from build123d import *

# Parameters (mm, degrees)
SKETCH_R     = 9
PAD_DEPTH    = 20
SKETCH002_W  = 12
SKETCH002_H  = 12
PAD001_DEPTH = 5
SKETCH003_R  = 2.6
POCKET_DEPTH = 25
CHAMFER_SIZE = 1


with BuildPart() as part:
    # Sketch → Pad (new body)
    with BuildSketch(Plane.XY):
        Circle(SKETCH_R)
    extrude(amount=PAD_DEPTH)

    # Sketch002 (on Face3 of Pad) → Pad001 (join)
    with BuildSketch(Plane.XY.offset(20)):
        Rectangle(SKETCH002_W, SKETCH002_H)
    extrude(amount=PAD001_DEPTH)

    # Sketch003 (on Face2 of Pad001) → Pocket (cut)
    with BuildSketch(Plane(origin=(0, 0, 0), x_dir=(1, 0, 0), z_dir=(0, 0, -1))):
        Circle(SKETCH003_R)
    extrude(amount=-POCKET_DEPTH, mode=Mode.SUBTRACT)

    # Chamfer
    chamfer_edges = [part.edges().sort_by_distance(p)[0] for p in [
        (-6, 0, 25),
        (0, -6, 25),
        (6, 0, 25),
        (0, 6, 25),
    ]]
    chamfer(chamfer_edges, length=CHAMFER_SIZE)


solid = part.part
For this review, take the finished solid that the model builds, in its own axes (mm). A direction names the side the tool comes from. Round coordinates to 2 decimals unless told otherwise and drop trailing zeros. Order: outer loops, then holes, each group sorted by start corner. A loop starts at its lowest first (then second) coordinate and runs counter-clockwise, first axis right, second up. Notation, with made-up numbers: M -4.75,17.25 L 30.25,17.25 A20 cw 30.25,50.25 Z; hole C -36,-11.75 d1. An arc over 180 degrees is marked long. Write each question's results on one line, items separated by ' | '. Start each with the question number.
1. Clearance check with flat-ended pins moving along their axes: pin 1 Ø5 at (x, z) = (-3, 20.5) entering from +Y; pin 2 Ø10 at (y, z) = (6, 8.5) entering from +X; pin 3 Ø1.5 at (x, z) = (5, 18) entering from -Y. State where each tip first meets the part, or that it passes through.
2. Draft analysis for pull direction X (two halves, no side actions). For faces 1 (the face through (-6, 0, 22)), 2 (the face through (-7, 1, 20)), 3 (the face through (-0.338, -2.578, 12.325)), 4 (the face through (-1.172, 8.923, 9.86)), state which applies: pulls with the +X half, pulls with the -X half, needs draft (parallel to the pull), parting line crosses it, or undercut.
3. To check wall thickness, follow L1, parallel to Y at x = 0, z = 18.75; L2, parallel to Z at x = 6.75, y = -4; L3, parallel to X at y = 0.75, z = 11.25. State the ranges of each line that lie inside material, in increasing order. Write a range as [from, to].
4. Add section D-D (y = 4.5). State the section outline as (x, z) points, then the cut area to 3 significant figures.
5. Tool access review of faces 5 (the face through (0, -6, 22)), 6 (the face through (2, -2, 0)), 7 (the face through (6, 0, 22)), 8 (the face through (0, 6, 22)), 9 (the face through (2, 2, 25)): name each direction out of +Z, -Z, +X, -X, +Y, -Y from which nothing blocks a thin tool from reaching the whole face with its end or side.
6. Add section A-A (x = 0). State the section outline as (y, z) points.
7. Add section C-C (z = 18.75). State the section outline as (x, y) points, then the cut area to 3 significant figures.
Output values:
1) pin 1: y = 8.98 | pin 2: x = 8.94 | pin 3: y = -7.93
2) face 1: pulls with the -X half | face 2: needs draft | face 3: undercut | face 4: parting line crosses it
3) L1: [-9, -2.6], [2.6, 9] | L2: [0, 20] | L3: [-8.97, -2.49], [2.49, 8.97]
4) outline: M -7.79,0 L 7.79,0 L 7.79,20 L 6,20 L 6,24 L 5,25 L -5,25 L -6,24 L -6,20 L -7.79,20 Z | area: 371 mm^2
5) face 5: +Z, +X, -X, -Y | face 6: -Z, +X, -X, +Y, -Y | face 7: +Z, +X, +Y, -Y | face 8: +Z, +X, -X, +Y | face 9: +Z, +X, -X, +Y, -Y
6) outline: M -9,0 L -2.6,0 L -2.6,25 L -5,25 L -6,24 L -6,20 L -9,20 Z; M 2.6,0 L 9,0 L 9,20 L 6,20 L 6,24 L 5,25 L 2.6,25 Z
7) outline: C 0,0 d18; hole C 0,0 d5.2 | area: 233 mm^2
